Work out the finished part from the listing and answer in its coordinate system (mm). Round coordinates to 2 decimals unless told otherwise and drop trailing zeros. Loops run counter-clockwise (first coordinate to the right, second up) from the corner with the lowest first, then second, coordinate; pieces in that order, holes last.
```python
from build123d import *

# Parameters (mm, degrees)
F1_DEPTH = 2


with BuildPart() as f1:
    # F0 (on Top) → F1 (new body)
    with BuildSketch(Plane.XY):
        Polygon((-30, 0), (-25, 0), (-20, 2.7), (0, 2.7), (0, 15), (-1, 15), (-1, 20), (-30, 2.1), align=None)
        Polygon((0, 15), (0, 2.7), (20, 2.7), (25, 0), (30, 0), (30, 2.1), (1, 20), (1, 15), align=None)
    extrude(amount=F1_DEPTH)


solid = f1.part
```
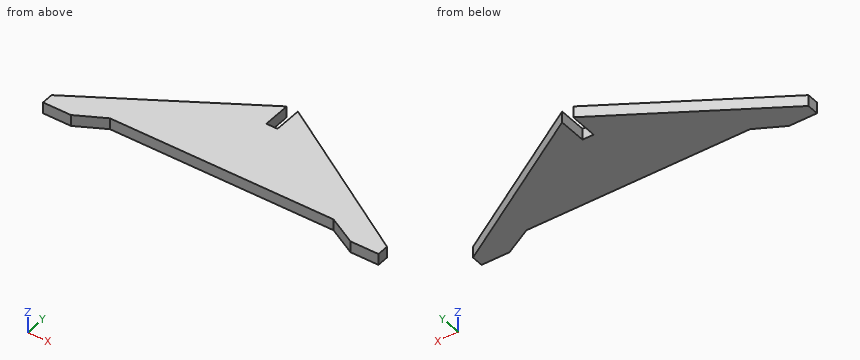
1. Find section A-A (y = 1.5). Write down the section's boundary in (x, z).
Answer key:
outline: (-30, 0) - (-22.22, 0) - (-22.22, 2) - (-30, 2) - close; (22.22, 0) - (30, 0) - (30, 2) - (22.22, 2) - close
2. Given pin 1 (1 mm diameter, centred on y = 18, z = 0.5, fed in from +X); pin 2 (0.6 mm diameter, centred on x = 0, z = 1.5, fed in from +Y); pin 3 (0.6 mm diameter, centred on x = -6, z = 1, fed in from -Y), each flat-ended and moving along its own axis, determine where each tip first touches the part or whether it passes through.
Answer key:
pin 1: stops at x = 5.05
pin 2: stops at y = 15
pin 3: stops at y = 2.7
3. Find section B-B (z = 1.35). Write down the section's boundary in (x, y).
Answer key:
outline: (-30, 0) - (-25, 0) - (-20, 2.7) - (20, 2.7) - (25, 0) - (30, 0) - (30, 2.1) - (1, 20) - (1, 15) - (-1, 15) - (-1, 20) - (-30, 2.1) - close
4. Find section D-D (y = 19). Write down the section's boundary in (x, z).
Answer key:
outline: (-2.62, 0) - (-1, 0) - (-1, 2) - (-2.62, 2) - close; (1, 0) - (2.62, 0) - (2.62, 2) - (1, 2) - close
5. Consider probe 1 along X at (y, z) = (1, 0.85); probe 2 along X at (y, z) = (18, 0.7); probe 3 along X at (y, z) = (9, 1.6). Determine where each line is inside the solid, lowest interval first.
Answer key:
probe 1: x = -30 to -23.15, 23.15 to 30
probe 2: x = -4.24 to -1, 1 to 4.24
probe 3: x = -18.82 to 18.82
6. Find section C-C (x = 15.5). Write down the section's boundary in (y, z), then the cut area to 3 significant figures.
Answer key:
outline: (2.7, 0) - (11.05, 0) - (11.05, 2) - (2.7, 2) - close
area: 16.7 mm2
